Design review of the part built by this model. Coordinates are the model's own, in mm. Face numbers are marked on the shaded views. A direction names the side the tool comes from. Give positions to 0.01 mm unless a question says otherwise; leave off trailing zeros. Write each loop counter-clockwise with the first axis right and the second up, starting at its lowest first coordinate (ties: lowest second). Pieces come first, ordered by that corner, then holes. Notation, with made-up numbers: M 3,7 L 34,7 A25 cw 34,31 Z; hole C -20.75,-9.75 d11. An arc over 180 degrees is marked long. Answer in a Markdown table with one row per item.
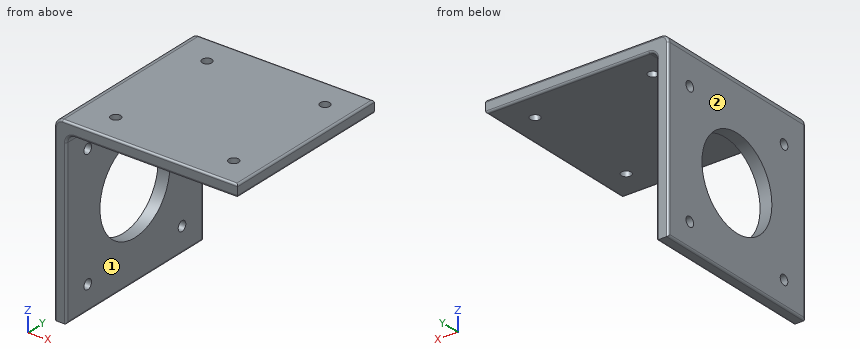
```python
from build123d import *

# Parameters (mm, degrees)
EXTRUDE_1_DEPTH     = 45
M3X0_5_1_D          = 2.5
FILLET_1_R          = 2
M3X0_5_2_D          = 2.5
FILLET_2_R          = 0.5
CUT_EXTRUDE_1_REACH = 69.032
SKETCH_6_R          = 11.5


with BuildPart() as part:
    # 草图1 → 拉伸-薄壁1 (new body)
    with BuildSketch(Plane(origin=(0, 0, 0), x_dir=(1, 0, 0), z_dir=(0, 1, 0))):
        Polygon((-24, 22.5), (-24, -24), (22.5, -24), (22.5, -21), (-21, -21), (-21, 22.5), align=None)
    extrude(amount=EXTRUDE_1_DEPTH)

    # M3x0.5 螺纹孔1 (through all)
    with Locations(Plane(origin=(-21, 38, 14.75), x_dir=(0, 0, 1), z_dir=(1, 0, 0))):
        with Locations((0, 0), (-31, 0), (-31, 31), (0, 31)):
            Hole(M3X0_5_1_D / 2)

    # 圆角1
    fillet_1_edges = [part.edges().sort_by_distance(p)[0] for p in [
        (-24, 22.5, 24),
        (-21, 22.5, 21),
    ]]
    fillet(fillet_1_edges, radius=FILLET_1_R)

    # M3x0.5 螺纹孔2 (through all)
    with Locations(Plane(origin=(-14.25, 37.5, 21), x_dir=(-1, 0, 0), z_dir=(0, 0, -1))):
        with Locations((0, 0), (0, -30), (-30, -30), (-30, 0)):
            Hole(M3X0_5_2_D / 2)

    # 圆角2
    fillet_2_edges = [part.edges().sort_by_distance(p)[0] for p in [
        (22.5, 22.5, 24),
        (-21, 45, -1.75),
        (-24, 45, -0.25),
        (0.25, 0, 24),
        (0.25, 45, 24),
        (1.75, 0, 21),
        (-23.414213562, 0, 23.414213562),
        (1.75, 45, 21),
        (-23.414213562, 45, 23.414213562),
        (-20.414213562, 0, 20.414213562),
        (-20.414213562, 45, 20.414213562),
        (-24, 0, -0.25),
        (-21, 0, -1.75),
        (-24, 22.5, -22.5),
        (-21, 22.5, -22.5),
        (22.5, 22.5, 21),
    ]]
    fillet(fillet_2_edges, radius=FILLET_2_R)

    # 草图6 → 切除-拉伸1 (cut, up to next)
    with BuildSketch(Plane(origin=(-21, 0, 0), x_dir=(0, 0, -1), z_dir=(1, 0, 0)), mode=Mode.PRIVATE) as cut_extrude_1_sk1:
        with Locations((0.75, 22.5)):
            Circle(SKETCH_6_R)
    cut_extrude_1_tool1 = extrude(cut_extrude_1_sk1.sketch, amount=-CUT_EXTRUDE_1_REACH, mode=Mode.PRIVATE) & part.part
    add(cut_extrude_1_tool1.solids().sort_by_distance((-21, 22.5, -0.75))[0], mode=Mode.SUBTRACT)


solid = part.part
```
1) Add section D-D (z = 14.75). Write out the cut boundary in (x, y).
Geometry says:
| item | result |
|---|---|
| outline | M -24,0.5 A0.5 ccw -23.5,0 L -21.5,0 A0.5 ccw -21,0.5 L -21,5.75 L -24,5.75 Z; M -24,8.25 L -21,8.25 L -21,36.75 L -24,36.75 Z; M -24,39.25 L -21,39.25 L -21,44.5 A0.5 ccw -21.5,45 L -23.5,45 A0.5 ccw -24,44.5 Z |
2) Add section A-A (z = -0.75). Write out the cut boundary in (x, y).
Geometry says:
| item | result |
|---|---|
| outline | M -24,0.5 A0.5 ccw -23.5,0 L -21.5,0 A0.5 ccw -21,0.5 L -21,11 L -24,11 Z; M -24,34 L -21,34 L -21,44.5 A0.5 ccw -21.5,45 L -23.5,45 A0.5 ccw -24,44.5 Z |
3) Insertion check: P1, Ø4, axis at y = 39.5, z = 1, coming from the +X side; P2, Ø4, axis at x = 15.75, y = 7.5, coming from the +Z side; P3, Ø6, axis at x = -15.5, z = -6, coming from the +Y side; P4, Ø12.5, axis at x = 6.5, y = 15.5, coming from the -Z side. Each pin has a flat end and moves straight along its axis. Give the tip position at first contact, or say it passes through.
Geometry says:
| item | result |
|---|---|
| P1 | x = -21 |
| P2 | z = 24 |
| P3 | through |
| P4 | z = 21 |
4) For the marked faces 1 and 2, list the 3-axis set-ups (+Z, -Z, +X, -X, +Y, -Y) from which the entire face can be reached by the end or side of a thin tool; tool diameter is ignored.
Geometry says:
| item | result |
|---|---|
| face 1 | -Z, +X, +Y, -Y |
| face 2 | +Z, -Z, -X, +Y, -Y |
5) Add section C-C (x = 15.75). Write out the cut boundary in (y, z), and give its area (3 significant figures).
Geometry says:
| item | result |
|---|---|
| outline | M 0,21.5 A0.5 ccw 0.5,21 L 6.25,21 L 6.25,24 L 0.5,24 A0.5 ccw 0,23.5 Z; M 8.75,21 L 36.25,21 L 36.25,24 L 8.75,24 Z; M 38.75,21 L 44.5,21 A0.5 ccw 45,21.5 L 45,23.5 A0.5 ccw 44.5,24 L 38.75,24 Z |
| area | 120 mm^2 |
6) To check wall thickness, follow probe 1 along Y at (x, z) = (15.75, 21.9); probe 2 along Y at (x, z) = (-23.4, 14.75); probe 3 along Z at (x, y) = (-23, 7). State the ranges of each line that lie inside material, in increasing order. Write a range as [from, to].
Geometry says:
| item | result |
|---|---|
| probe 1 | [0, 6.25], [8.75, 36.25], [38.75, 45] |
| probe 2 | [0, 5.75], [8.25, 36.75], [39.25, 45] |
| probe 3 | [-22.5, -17.5], [-15, 13.5], [16, 23.73] |
7) Add section B-B (y = 22.5). Write out the cut boundary in (x, z), and give its area (3 significant figures).
Geometry says:
| item | result |
|---|---|
| outline | M -24,-22 A0.5 ccw -23.5,-22.5 L -21.5,-22.5 A0.5 ccw -21,-22 L -21,-12.25 L -24,-12.25 Z; M -24,10.75 L -21,10.75 L -21,19 A2 cw -19,21 L 22,21 A0.5 ccw 22.5,21.5 L 22.5,23.5 A0.5 ccw 22,24 L -22,24 A2 ccw -24,22 Z |
| area | 201 mm^2 |
